```python
from build123d import *

# Parameters (mm, degrees)
BOSS_EXTRUDE1_DEPTH      = 2
SKETCH2_W                = 2
SKETCH2_H                = 60
BOSS_EXTRUDE2_DEPTH      = 55
SKETCH3_R                = 5
CUT_EXTRUDE1_DEPTH       = 283
SKETCH4_R                = 2.5
CUT_EXTRUDE2_DEPTH       = 283
SKETCH9_W                = 230
SKETCH9_H                = 50
BOSS_EXTRUDE3_DEPTH      = 2
SKETCH13_W               = 230
SKETCH13_H               = 10
BOSS_EXTRUDE6_DEPTH      = 20
CUT_EXTRUDE9_START       = -230
CUT_EXTRUDE9_DEPTH       = 230
CUT_EXTRUDE14_DEPTH      = 180.947909129
CUT_EXTRUDE14_DEPTH_BACK = 180.947909129
BOSS_EXTRUDE8_DEPTH      = 60
SKETCH38_W               = 90
SKETCH38_H               = 5
BOSS_EXTRUDE9_DEPTH      = 50
CUT_EXTRUDE15_DEPTH      = 50
CUT_EXTRUDE16_DEPTH      = 152.492574075
CUT_EXTRUDE16_DEPTH_BACK = 152.492574075
BOSS_EXTRUDE10_DEPTH     = 90


# Read off the part's stored shape, not the designer's step: Cut-Extrude9
with BuildPart() as part:
    # Sketch1 → Boss-Extrude1 (new body)
    with BuildSketch(Plane(origin=(0, 0, 0), x_dir=(1, 0, 0), z_dir=(0, 1, 0))):
        Polygon((115, 50), (115, 80), (-115, 80), (-115, 50), (-115, -50), (-115, -75), (115, -75), (115, -50), align=None)
    extrude(amount=BOSS_EXTRUDE1_DEPTH)

    # Sketch2 → Boss-Extrude2 (add)
    with BuildSketch(Plane(origin=(0, 2, 0), x_dir=(1, 0, 0), z_dir=(0, 1, 0))):
        with Locations((-114, 0)):
            Rectangle(SKETCH2_W, SKETCH2_H)
        with Locations((114, 0)):
            Rectangle(SKETCH2_W, SKETCH2_H)
    extrude(amount=BOSS_EXTRUDE2_DEPTH)

    # Sketch3 → Cut-Extrude1 (cut)
    with BuildSketch(Plane.ZY.offset(115)):
        with Locations((0, 29.5)):
            Circle(SKETCH3_R)
    extrude(amount=-CUT_EXTRUDE1_DEPTH, mode=Mode.SUBTRACT)

    # Sketch4 → Cut-Extrude2 (cut)
    with BuildSketch(Plane.ZY.offset(115)):
        with Locations((-22.5, 29.5)):
            Circle(SKETCH4_R)
        with Locations((22.5, 29.5)):
            Circle(SKETCH4_R)
    extrude(amount=-CUT_EXTRUDE2_DEPTH, mode=Mode.SUBTRACT)

    # Sketch9 → Boss-Extrude3 (add)
    with BuildSketch(Plane(origin=(0, 2, 0), x_dir=(1, 0, 0), z_dir=(0, 1, 0))):
        with Locations((0, 105)):
            Rectangle(SKETCH9_W, SKETCH9_H)
    extrude(amount=-BOSS_EXTRUDE3_DEPTH)

    # Sketch13 → Boss-Extrude6 (add)
    with BuildSketch(Plane.XZ):
        with Locations((0, -125)):
            Rectangle(SKETCH13_W, SKETCH13_H)
    extrude(amount=BOSS_EXTRUDE6_DEPTH)

    # Cut-Extrude9 outline → Cut-Extrude9 (cut)
    with BuildSketch(Plane(origin=(115, 0, 0), x_dir=(0, 0, -1), z_dir=(1, 0, 0)).offset(CUT_EXTRUDE9_START)):
        with BuildLine():
            Line((-30, 57), (-30, 29.5))
            ThreePointArc((-30, 29.5), (0, 49.5), (30, 29.5))
            Line((30, 29.5), (30, 57))
            Line((30, 57), (-30, 57))
        make_face()
    extrude(amount=CUT_EXTRUDE9_DEPTH, mode=Mode.SUBTRACT)

    # Sketch34 → Cut-Extrude14 (cut, two sides: drawn at the far end of the back side and taken through both)
    with BuildSketch(Plane(origin=(0, 2, 0), x_dir=(1, 0, 0), z_dir=(0, 1, 0)).offset(-CUT_EXTRUDE14_DEPTH_BACK)):
        Polygon((685.357029045, 85), (115, 85), (-115, 85), (-685.357029045, 85), (-685.357029045, 1225.71405809), (685.357029045, 1225.71405809), align=None)
    extrude(amount=CUT_EXTRUDE14_DEPTH + CUT_EXTRUDE14_DEPTH_BACK, mode=Mode.SUBTRACT)

    # Sketch37 → Boss-Extrude8 (add)
    with BuildSketch(Plane(origin=(0, 0, -30), x_dir=(-1, 0, 0), z_dir=(0, 0, -1))):
        with BuildLine():
            Line((-103, 2), (-113, 2))
            Line((-113, 2), (-113, 12))
            ThreePointArc((-113, 12), (-110.071067812, 4.928932188), (-103, 2))
        make_face()
        with BuildLine():
            Line((103, 2), (113, 2))
            Line((113, 2), (113, 12))
            ThreePointArc((113, 12), (110.071067812, 4.928932188), (103, 2))
        make_face()
    extrude(amount=-BOSS_EXTRUDE8_DEPTH)

    # Sketch38 → Boss-Extrude9 (add)
    with BuildSketch(Plane(origin=(0, 2, 0), x_dir=(1, 0, 0), z_dir=(0, 1, 0))):
        with Locations((0, -50)):
            Rectangle(SKETCH38_W, SKETCH38_H)
    extrude(amount=BOSS_EXTRUDE9_DEPTH)

    # Sketch39 → Cut-Extrude15 (cut)
    with BuildSketch(Plane.XY.offset(52.5)):
        with BuildLine():
            Line((0, 52), (-20, 52))
            Line((-20, 52), (-20, 22))
            ThreePointArc((-20, 22), (-17.071067812, 14.928932188), (-10, 12))
            Line((-10, 12), (10, 12))
            ThreePointArc((10, 12), (17.071067812, 14.928932188), (20, 22))
            Line((20, 22), (20, 52))
            Line((20, 52), (0, 52))
        make_face()
        with BuildLine():
            ThreePointArc((27.189233611, 19.321452148), (30, 32), (27.189233611, 44.678547852))
            ThreePointArc((27.189233611, 44.678547852), (28.398457424, 48.000862974), (31.720772546, 46.791639161))
            ThreePointArc((31.720772546, 46.791639161), (35, 32), (31.720772546, 17.208360839))
            ThreePointArc((31.720772546, 17.208360839), (28.398457424, 15.999137026), (27.189233611, 19.321452148))
        make_face()
        with BuildLine():
            ThreePointArc((-27.189233611, 19.321452148), (-28.398457424, 15.999137026), (-31.720772546, 17.208360839))
            ThreePointArc((-31.720772546, 17.208360839), (-35, 32), (-31.720772546, 46.791639161))
            ThreePointArc((-31.720772546, 46.791639161), (-28.398457424, 48.000862974), (-27.189233611, 44.678547852))
            ThreePointArc((-27.189233611, 44.678547852), (-30, 32), (-27.189233611, 19.321452148))
        make_face()
    extrude(amount=-CUT_EXTRUDE15_DEPTH, mode=Mode.SUBTRACT)

    # Sketch40 → Cut-Extrude16 (cut, two sides: drawn at the far end of the back side and taken through both)
    with BuildSketch(Plane(origin=(0, 2, 0), x_dir=(1, 0, 0), z_dir=(0, 1, 0)).offset(-CUT_EXTRUDE16_DEPTH_BACK)):
        Polygon((-614.144418911, 130.439277507), (-115, -30), (-45, -52.5), (45, -52.5), (115, -30), (614.144418911, 130.439277507), (614.144418911, -918.151992143), (-614.144418911, -918.151992143), align=None)
    extrude(amount=CUT_EXTRUDE16_DEPTH + CUT_EXTRUDE16_DEPTH_BACK, mode=Mode.SUBTRACT)

    # Sketch41 → Boss-Extrude10 (add)
    with BuildSketch(Plane.ZY.offset(45)):
        with BuildLine():
            Line((37.5, 2), (47.5, 2))
            Line((47.5, 2), (47.5, 12))
            ThreePointArc((47.5, 12), (44.571067812, 4.928932188), (37.5, 2))
        make_face()
    extrude(amount=-BOSS_EXTRUDE10_DEPTH)


solid = part.part
```
CAD build for the part. Positions are in the model's coordinates, mm. A direction names the side the tool comes from. Round coordinates to 2 decimals unless told otherwise and drop trailing zeros. Loops run counter-clockwise (first coordinate to the right, second up) from the corner with the lowest first, then second, coordinate; pieces in that order, holes last. Notation, with made-up numbers: M 8.25,37 L 19.25,37 A14 cw 19.25,55 Z; hole C -34,7 d6. An arc over 180 degrees is marked long. Return JSON: item names as keys, results as strings. Group by question number.
(1) Saw through at D-D, the plane y = 40. List the corners of the cut face in (x, z).
(2) Tool access for faces 5 (the flat face through (45, 25, 49)), 6 (the cylindrical face through (-30, 32, 50)), 7 (the cylindrical face through (-114.01, 24.62, -1.08)), 8 (the flat face through (-113.4, 11.7, -30)), 9 (the flat face through (20, 37, 50)): list every direction of +Z, -Z, +X, -X, +Y, -Y with a clear straight run to the whole face (end or side of a thin tool).
(3) Wall check: probe 1 along X at (y, z) = (31, -15); probe 2 along Y at (x, z) = (114, 0); probe 3 along X at (y, z) = (11, 21). Give the ranges that are in metal, low to high. Write a range as [from, to].
(4) Saw through at B-B, the plane y = 6. List the corners of the cut face in (x, z).
(5) Saw through at C-C, the plane x = -24.5. List the corners of the cut face in (y, z), and give its area (3 significant figures).
(6) Mould opens along X. For faces 1 (the cylindrical face through (16.99, 14.85, 50.04)), 2 (the flat face through (-1, 8, 52.5)), 3 (the flat face through (-115, 20, -3)), 4 (the flat face through (-20, 37, 50)) say: +X half, -X half, draft (parallel to the pull), parting line (faces both ways), or undercut.
(7) Drop flat-ended pins along their axis: P1, Ø13, axis at x = -111, y = 14, coming from the +Z side; P2, Ø9, axis at y = 29.5, z = 0, coming from the -X side; P3, Ø8, axis at y = 29.5, z = -22.5, coming from the -X side; P4, Ø4, axis at y = 40, z = 49.5, coming from the +X side. Give the stop position or say it passes through.
(8) Saw through at A-A, the plane z = 0. List the corners of the cut face in (x, y).
Answer list:
{
 "1": {"outline": "M -115,-22.96 L -113,-22.96 L -113,22.96 L -115,22.96 Z; M -45,47.5 L -34.07,47.5 L -34.07,52.5 L -45,52.5 Z; M -28.91,47.5 L -20,47.5 L -20,52.5 L -28.91,52.5 Z; M 20,47.5 L 28.91,47.5 L 28.91,52.5 L 20,52.5 Z; M 34.07,47.5 L 45,47.5 L 45,52.5 L 34.07,52.5 Z; M 113,-22.96 L 115,-22.96 L 115,22.96 L 113,22.96 Z"},
 "2": {"face 5": "+Z, -Z, +X, +Y", "face 6": "+Z, -Z", "face 7": "+X, -X", "face 8": "-Z, +X, -X, +Y", "face 9": "+Z, -Z, +Y"},
 "3": {"probe 1": "[-115, -113], [113, 115]", "probe 2": "[0, 24.5], [34.5, 49.5]", "probe 3": "[-115, -112.95], [112.95, 115]"},
 "4": {"outline": "M -115,-30 L -111,-30 L -111,30 L -115,30 Z; M -45,45.5 L 45,45.5 L 45,52.5 L -45,52.5 Z; M 111,-30 L 115,-30 L 115,30 L 111,30 Z"},
 "5": {"outline": "M 0,-85 L 2,-85 L 2,37.5 A10 cw 12,47.5 L 52,47.5 L 52,52.5 L 0,52.5 Z", "area": "546 mm2"},
 "6": {"face 1": "undercut", "face 2": "draft", "face 3": "-X half", "face 4": "undercut"},
 "7": {"P1": "z = 30", "P2": "through", "P3": "x = -115", "P4": "x = 45"},
 "8": {"outline": "M -115,0 L 115,0 L 115,24.5 L 113,24.5 L 113,12 A10 cw 103,2 L -103,2 A10 cw -113,12 L -113,24.5 L -115,24.5 Z; M -115,34.5 L -113,34.5 L -113,49.5 L -115,49.5 Z; M 113,34.5 L 115,34.5 L 115,49.5 L 113,49.5 Z"}
}
